from build123d import *

# Parameters (mm, degrees)
SKETCH1_W           = 66
SKETCH1_H           = 53.2
SKETCH1_R           = 1
SKETCH1_R_2         = 0.98333
SKETCH1_R_3         = 1.011270727
BOSS_EXTRUDE1_DEPTH = 1.5
SKETCH2_W           = 5
SKETCH2_H           = 5
BOSS_EXTRUDE2_DEPTH = 2
FILLET1_R           = 1
FILLET2_R           = 2.5
SKETCH3_R           = 2
BOSS_EXTRUDE3_DEPTH = 3
SKETCH4_R           = 1
CUT_EXTRUDE1_DEPTH  = 384.370615534
SKETCH5_W           = 24
SKETCH5_H           = 10
CUT_EXTRUDE2_DEPTH  = 3
FILLET3_R           = 1


with BuildPart() as part:
    # Sketch1 → Boss-Extrude1 (new body)
    with BuildSketch(Plane.XY.offset(10)):
        with Locations((177.963936399, 293.439054482)):
            Rectangle(SKETCH1_W, SKETCH1_H)
        with Locations((161.947495, 317.06050799)):
            Circle(SKETCH1_R, mode=Mode.SUBTRACT)
        with Locations((193.956452611, 317.06050799)):
            Circle(SKETCH1_R, mode=Mode.SUBTRACT)
        with Locations((174.997800233, 314.982847455)):
            Circle(SKETCH1_R, mode=Mode.SUBTRACT)
        with Locations((181.100928053, 314.982847455)):
            Circle(SKETCH1_R, mode=Mode.SUBTRACT)
        with Locations((173.997800233, 290.965333254)):
            Circle(SKETCH1_R_2, mode=Mode.SUBTRACT)
        with Locations((181.983306885, 290.965333254)):
            Circle(SKETCH1_R, mode=Mode.SUBTRACT)
        with Locations((161.947495, 286.962677261)):
            Circle(SKETCH1_R, mode=Mode.SUBTRACT)
        with Locations((193.956452611, 286.962677261)):
            Circle(SKETCH1_R, mode=Mode.SUBTRACT)
        with Locations((162.947495, 268.970540104)):
            Circle(SKETCH1_R, mode=Mode.SUBTRACT)
        with Locations((192.956452611, 268.970540104)):
            Circle(SKETCH1_R_3, mode=Mode.SUBTRACT)
        with Locations((208.084556857, 269.981810832)):
            Circle(SKETCH1_R, mode=Mode.SUBTRACT)
        with Locations((147.966567684, 269.970540104)):
            Circle(SKETCH1_R, mode=Mode.SUBTRACT)
    extrude(amount=BOSS_EXTRUDE1_DEPTH)

    # Sketch2 → Boss-Extrude2 (add)
    with BuildSketch(Plane.XY.offset(11.5)):
        with Locations((195.50417089, 308.439334712)):
            Rectangle(SKETCH2_W, SKETCH2_H)
        with Locations((160.50417089, 308.439334712)):
            Rectangle(SKETCH2_W, SKETCH2_H)
        with Locations((195.50417089, 273.439334712)):
            Rectangle(SKETCH2_W, SKETCH2_H)
        with Locations((160.50417089, 273.439334712)):
            Rectangle(SKETCH2_W, SKETCH2_H)
    extrude(amount=BOSS_EXTRUDE2_DEPTH)

    # Fillet1
    fillet1_edges = [part.edges().sort_by_distance(p)[0] for p in [
        (163.00417089, 275.939334712, 12.5),
        (158.00417089, 275.939334712, 12.5),
        (158.00417089, 270.939334712, 12.5),
        (163.00417089, 270.939334712, 12.5),
        (158.00417089, 310.939334712, 12.5),
        (158.00417089, 305.939334712, 12.5),
        (163.00417089, 305.939334712, 12.5),
        (163.00417089, 310.939334712, 12.5),
        (198.00417089, 310.939334712, 12.5),
        (193.00417089, 310.939334712, 12.5),
        (193.00417089, 305.939334712, 12.5),
        (198.00417089, 305.939334712, 12.5),
        (198.00417089, 275.939334712, 12.5),
        (193.00417089, 275.939334712, 12.5),
        (193.00417089, 270.939334712, 12.5),
        (198.00417089, 270.939334712, 12.5),
    ]]
    fillet(fillet1_edges, radius=FILLET1_R)

    # Fillet2
    fillet2_edges = [part.edges().sort_by_distance(p)[0] for p in [
        (144.963936399, 320.039054482, 10.75),
        (210.963936399, 320.039054482, 10.75),
        (210.963936399, 266.839054482, 10.75),
        (144.963936399, 266.839054482, 10.75),
    ]]
    fillet(fillet2_edges, radius=FILLET2_R)

    # Sketch3 → Boss-Extrude3 (add)
    with BuildSketch(Plane.XY.offset(13.5)):
        with Locations(Location((159.986771392, 308.993272747, 0), (0, 0, 187.563213286))):
            Circle(SKETCH3_R)
        with Locations(Location((195.986771392, 308.993272747, 0), (0, 0, 103.336783262))):
            Circle(SKETCH3_R)
        with Locations((195.986771392, 272.993272747)):
            Circle(SKETCH3_R)
        with Locations(Location((159.986771392, 272.993272747, 0), (0, 0, 187.563213286))):
            Circle(SKETCH3_R)
    extrude(amount=BOSS_EXTRUDE3_DEPTH)

    # Sketch4 → Cut-Extrude1 (cut, through all)
    with BuildSketch(Plane.XY.offset(16.5)):
        with Locations((159.979889168, 308.96706871)):
            Circle(SKETCH4_R)
        with Locations((195.979889168, 308.96706871)):
            Circle(SKETCH4_R)
        with Locations((195.979889168, 272.96706871)):
            Circle(SKETCH4_R)
        with Locations((159.979889168, 272.96706871)):
            Circle(SKETCH4_R)
    extrude(amount=-CUT_EXTRUDE1_DEPTH, mode=Mode.SUBTRACT)

    # Sketch5 → Cut-Extrude2 (cut)
    with BuildSketch(Plane.XY.offset(11.5)):
        Polygon((199.987014771, 283.959443526), (207.987014771, 283.959443526), (207.970870972, 274.289443526), (204.987014771, 271.959443526), (199.987014771, 271.959443526), align=None)
        Polygon((150.940858028, 271.959443526), (155.940858028, 271.959443526), (155.940858028, 283.959443526), (147.940858028, 283.959443526), (147.957001827, 274.289443526), align=None)
        with Locations((178.030567575, 275.960587895)):
            Rectangle(SKETCH5_W, SKETCH5_H)
    extrude(amount=-CUT_EXTRUDE2_DEPTH, mode=Mode.SUBTRACT)

    # Fillet3
    fillet3_edges = [part.edges().sort_by_distance(p)[0] for p in [
        (199.987014771, 271.959443526, 10.75),
        (199.987014771, 283.959443526, 10.75),
        (207.987014771, 283.959443526, 10.75),
        (207.970870972, 274.289443526, 10.75),
        (204.987014771, 271.959443526, 10.75),
        (150.940858028, 271.959443526, 10.75),
        (147.957001827, 274.289443526, 10.75),
        (147.940858028, 283.959443526, 10.75),
        (155.940858028, 283.959443526, 10.75),
        (155.940858028, 271.959443526, 10.75),
        (166.030567575, 270.960587895, 10.75),
        (166.030567575, 280.960587895, 10.75),
        (190.030567575, 280.960587895, 10.75),
        (190.030567575, 270.960587895, 10.75),
    ]]
    fillet(fillet3_edges, radius=FILLET3_R)


solid = part.part
The listing builds one solid part. Answer for the finished solid, in the listing's coordinates (mm). A direction names the side the tool comes from. Coordinates: 2 decimals unless noted, no trailing zeros. Write each loop counter-clockwise with the first axis right and the second up, starting at its lowest first coordinate (ties: lowest second). Pieces come first, ordered by that corner, then holes. Notation, with made-up numbers: M -8,-32 L 35,-32 A23 cw 35,-24 Z; hole C 16,77 d2. An arc over 180 degrees is marked long. Put each result on its own line as item: value. Start each with the question number.
1. Which of the six approach directions +Z, -Z, +X, -X, +Y, -Y give full straight-line access (tool end or side, diameter ignored) to faces 4 (the flat face through (194, 307, 13.5)), 5 (the flat face through (160, 275.939, 12)), 6 (the flat face through (163.004, 308, 12)), 7 (the flat face through (198.004, 308, 12)), 8 (the flat face through (203, 271.959, 11))?
2. For a pull along Y with two mould halves and no side action, classify faces 1 (the cylindrical face through (180.884, 314.007, 10.74)), 2 (the flat face through (158.004, 308, 12)), 3 (the cylindrical face through (210.21, 267.55, 10.76)) as pulls with the +Y half, pulls with the -Y half, needs draft (parallel to the pull), parting line crosses it, or undercut.
3. Consider line 1 (Y direction, x = 194, z = 11); line 2 (X direction, y = 274.5, z = 12.5); line 3 (Y direction, x = 148.5, z = 11). Determine where each line is inside the solid, lowest interval first. Write a range as from..to.
4. A cutting plane is placed at D-D on y = 302.5. Write down the section's boundary in (x, z), then the cut area to 3 significant figures.
5. A cutting plane is placed at B-B on z = 15. Write down the section's boundary in (x, y), then the cut area to 3 significant figures.
6. Flat-ended cylindrical pins translate along their axes: P1, Ø8, axis at x = 158, y = 299.5, coming from the +Z side; P2, Ø1.6, axis at x = 195.5, z = 12.5, coming from the +Y side; P3, Ø2, axis at y = 275.5, z = 14, coming from the -X side. Find the tip coordinate at first contact, or state that the pin passes through.
7. A cutting plane is placed at A-A on x = 170.5. Write down the section's boundary in (y, z), then the cut area to 3 significant figures.
8. A cutting plane is placed at C-C on x = 206. Write down the section's boundary in (y, z), then the cut area to 3 significant figures.
Resolved:
1. face 4: +Z
1. face 5: +Z, +X, -X
1. face 6: +Z, +Y, -Y
1. face 7: +Z, +X, +Y, -Y
1. face 8: +Z, -Z
2. face 1: undercut
2. face 2: needs draft
2. face 3: pulls with the -Y half
3. line 1: y = 266.84..285.96, 287.96..316.06, 318.06..320.04
3. line 2: x = 158..163, 193..198
3. line 3: y = 266.84..269.12, 270.82..273.87, 283.86..320.04
4. outline: M 144.96,10 L 210.96,10 L 210.96,11.5 L 144.96,11.5 Z
4. area: 99.0 mm2
5. outline: C 159.99,272.99 d4; C 159.99,308.99 d4; C 195.99,272.99 d4; C 195.99,308.99 d4; hole C 159.98,272.97 d2; hole C 159.98,308.97 d2; hole C 195.98,272.97 d2; hole C 195.98,308.97 d2
5. area: 37.7 mm2
6. P1: stops at z = 11.5
6. P2: stops at y = 310.94
6. P3: stops at x = 158
7. outline: M 266.84,10 L 270.96,10 L 270.96,11.5 L 266.84,11.5 Z; M 280.96,10 L 320.04,10 L 320.04,11.5 L 280.96,11.5 Z
7. area: 64.8 mm2
8. outline: M 266.84,10 L 272.75,10 L 272.75,11.5 L 266.84,11.5 Z; M 283.96,10 L 320.04,10 L 320.04,11.5 L 283.96,11.5 Z
8. area: 63.0 mm2
